Autodesk Inventor part; units mm, degrees
ref_plane "YZ Plane" through (0, 0, 0) normal (1, 0, 0) x (0, 1, 0)
ref_plane "XZ Plane" through (0, 0, 0) normal (0, 1, 0) x (-1, 0, 0)
ref_plane "XY Plane" through (0, 0, 0) normal (0, 0, 1) x (1, 0, 0)
sketch "Sketch1" plane through (0, 0, 0) normal (0, 1, 0) x (-1, 0, 0)
  line L0 (0, 0) -> (16, 0)
  line L1 (16, 0) -> (16, -28)
  line L2 (16, -28) -> (0, -28)
  line L3 (0, -28) -> (0, 0)
  dimension "d0" = 16
  dimension "d1" = 28
extrude "Extrusion1" add sketch "Sketch1" along normal blind 3
sketch "Sketch2" plane through (0, 3, 0) normal (0, 1, 0) x (1, 0, 0)
  circle A0 centre (-3.3, 24.7) radius 2
  circle A1 centre (-12.7, 3.3) radius 2
  line L0 (0, 28) -> (-16, 28)
  line L1 (0, 0) -> (0, 28)
  line L2 (-16, 28) -> (-16, 0)
  line L3 (-16, 0) -> (0, 0)
  dimension "d4" = 4
  dimension "d5" = 4
  dimension "d6" = 3.3
  dimension "d7" = 3.3
  dimension "d8" = 3.3
  dimension "d9" = 3.3
extrude "Extrusion2" cut sketch "Sketch2" against normal blind 3.3 contours A0 | A1
sketch "Sketch10" plane through (0, 3, 0) normal (0, 1, 0) x (1, 0, 0)
  line L0 (-16, 28) -> (-16, 0)
  line L1 (-16, 14) -> (-16, 4)
  line L2 (-16, 4) -> (-24, 4)
  line L3 (-16, 0) -> (0, 0)
  line L4 (-16, 0) -> (-31, 0)
  line L5 (-31, 0) -> (-31, 9)
  line L6 (-31, 9) -> (-16, 9)
  line L7 (-16, 9) -> (-16, 0)
  line L8 (0, 28) -> (-16, 28)
  line L9 (-16, 28) -> (-31, 28)
  line L10 (-31, 28) -> (-31, 19)
  line L11 (-31, 19) -> (-16, 19)
  line L12 (-16, 19) -> (-16, 28)
  dimension "d52" = 10
  dimension "d53" = 8
  dimension "d54" = 15
  dimension "d55" = 9
  dimension "d56" = 15
  dimension "d57" = 9
extrude "Extrusion9" add sketch "Sketch10" against normal blind 6
sketch "Sketch11" plane through (0, 3, 0) normal (0, 1, 0) x (1, 0, 0)
  circle A0 centre (-23, 4) radius 3
  circle A1 centre (-23, 24) radius 3
  line L0 (-31, 0) -> (0, 0)
  line L1 (-31, 9) -> (-31, 0)
  line L2 (-31, 28) -> (-31, 19)
  dimension "d60" = 6
  dimension "d61" = 6
  dimension "d62" = 4
  dimension "d63" = 20
  dimension "d64" = 8
  dimension "d65" = 8
extrude "Extrusion10" cut sketch "Sketch11" against normal through all
sketch "Sketch12" plane through (0, -3, 0) normal (0, -1, 0) x (1, 0, 0)
  line L0 (-16, -9) -> (-31, -9)
  line L1 (-16, -9) -> (-18, -9)
  line L2 (-18, -9) -> (-18, 0)
  line L3 (-18, 0) -> (-16, 0)
  line L4 (-16, 0) -> (-16, -9)
  point P0 (0, 0)
  dimension "d68" = 2
  dimension "d69" = 9
extrude "Extrusion11" cut sketch "Sketch12" against normal blind 3
fillet "Fillet1" radius 2 2 edges at (-16, 0, -23.5) (-18, 0, -4.5)
fillet "Fillet2" radius 2 3 edges at (-15.5, 3, 0) (0, 3, -14) (-15.5, 3, -28)
fillet "Fillet3" radius 2 8 edges at (-31, 2.4142, -27.4142) (-31, -1, -28) (-31, 3, -22.5) (-23.5, 3, -19) (-23.5, 3, -9) (-31, 2.4142, -0.5858) (-31, -1, 0) (-31, 3, -5.5)
fillet "Fillet4" radius 2 2 edges at (-16, 3, -8) (-16, 3, -20)
equation "\"d10\" = d7"
properties part number "Limit_SwitchMount"
Input: part model. Units: mm. Frame: model coordinates. A direction names the side the tool comes from. Coordinates: 2 decimals unless noted, no trailing zeros. Loops run counter-clockwise (first coordinate to the right, second up) from the corner with the lowest first, then second, coordinate; pieces in that order, holes last.
Q1. Set-up query: faces 1 (the face through (-24, -1, -9)), 2 (the face through (-18, -2.5, -4.6)), 3 (the face through (-22.38, 2.43, -19.6)), 4 (the face through (-16, -2.5, -23.6)). Return all of +Z, -Z, +X, -X, +Y, -Y with unobstructed straight access to the full face (end or side cutting, diameter ignored); none if empty.
Q2. Material intervals for line 1 (Z direction, x = -12.7, y = 0.7); line 2 (Z direction, x = -3.3, y = 1.15); line 3 (X direction, y = 2.3, z = -24.7), sorted ascending.
Q3. Cut plane D-D (z = -24). Output: boundary loops of the cut face in (x, y), then the cut area to 3 significant figures.
Q4. Cut plane A-A (y = -2.5). Output: boundary loops of the cut face in (x, z).
Q5. Cut plane C-C (y = 0.5). Output: boundary loops of the cut face in (x, z).
Q6. Cut plane B-B (x = -27). Output: boundary loops of the cut face in (y, z).
Q7. Draft query along Z for faces 5 (the face through (-30.4, -0.97, -27.43)), 6 (the face through (-26, 0, -4)), 7 (the face through (-15.43, -0.6, -23.56)). Return one class per face: +Z half, -Z half, draft (parallel to the pull), parting line (faces both ways), or undercut.
Q8. Contact query for flat-ended pins moving along their axis: pin 1 (6.5 mm diameter, centred on x = -3.3, z = -24.7, fed in from -Y); pin 2 (1.1 mm diameter, centred on y = 0.5, z = -14, fed in from -X); pin 3 (6 mm diameter, centred on x = -12, z = -24.5, fed in from -Y). Output: stop coordinate, or through.
Working result:
1. face 1: -X, +Y, -Y
1. face 2: +Z, +X, -Y
1. face 3: -X, +Y
1. face 4: +Z, -Z, +X, -Y
2. line 1: z = -28 to -5.3, -1.3 to 0
2. line 2: z = -27.99 to -26.7, -22.7 to -0.01
2. line 3: x = -30.52 to -25.92, -20.08 to -5.3, -1.3 to -0.48
3. outline: (-31, -3) - (-26, -3) - (-26, 3) - (-29, 3) arc R2 ccw to (-31, 1) - close; (-20, -3) - (-16, -3) - (-16, -2) arc R2 cw to (-14, 0) - (-5.17, 0) - (-5.17, 3) - (-20, 3) - close; (-1.43, 0) - (0, 0) - (0, 1) arc R2 ccw to (-1.43, 2.92) - close
3. area: 89.9 mm2
4. outline: (-31, -26) arc R2 ccw to (-29, -28) - (-16, -28) - (-16, -19) - (-31, -19) - close; (-31, -9) - (-18, -9) - (-18, 0) - (-29, 0) arc R2 ccw to (-31, -2) - close; hole circle Ø6 at (-23, -24); hole circle Ø6 at (-23, -4)
5. outline: (-31, -26) arc R2 ccw to (-29, -28) - (0, -28) - (0, 0) - (-29, 0) arc R2 ccw to (-31, -2) - (-31, -9) - (-16, -9) - (-16, -19) - (-31, -19) - close; hole circle Ø6 at (-23, -24); hole circle Ø6 at (-23, -4); hole circle Ø4 at (-12.7, -3.3); hole circle Ø4 at (-3.3, -24.7)
6. outline: (-3, -28) - (1, -28) arc R2 ccw to (3, -26) - (3, -21) arc R2 ccw to (1, -19) - (-3, -19) - close; (-3, -9) - (1, -9) arc R2 ccw to (3, -7) - (3, -2) arc R2 ccw to (1, 0) - (-3, 0) - close
7. face 5: -Z half
7. face 6: undercut
7. face 7: draft
8. pin 1: stops at y = 0
8. pin 2: stops at x = -16
8. pin 3: stops at y = -0.27
